Check sheet for the modelled part. Datum: model origin and axes. Units: mm. Round coordinates to 2 decimals unless told otherwise and drop trailing zeros. Write each loop counter-clockwise with the first axis right and the second up, starting at its lowest first coordinate (ties: lowest second). Pieces come first, ordered by that corner, then holes.
Item 1: Cross-section at A-A on x = -29. Enter the section's corners in (y, z), plus the area to 3 significant figures.
Item 2: Material ranges on line 1 (Z direction, x = 19, y = 0.75); line 2 (Z direction, x = -29, y = 0.35); line 3 (X direction, y = 0.7, z = 23), recorded low to high.
Item 3: Go/stop test with a flat-tipped pin: pin 1 Ø5 at (x, z) = (-29, -23) entering from +Y. Record where the tip stops, or that it passes through.
Item 4: Cross-section at B-B on x = 19. Enter the section's corners in (y, z), plus the area to 3 significant figures.
from build123d import *

# Parameters (mm, degrees)
SKETCH1_W                    = 85
SKETCH1_H                    = 56
BOSS_EXTRUDE1_DEPTH          = 3
M2_CLEARANCE_HOLE1_D         = 2.2
M2_CLEARANCE_HOLE1_DEPTH     = 5
M2_CLEARANCE_HOLE1_TIP       = 0.660946681
FILLET1_R                    = 3
CSK_FOR_M3_SFHCS1_AT_2_COUNT = 2
CSK_FOR_M3_SFHCS1_AT_2_PITCH = 74.027022093
CSK_FOR_M3_SFHCS1_AT_3_COUNT = 2
CSK_FOR_M3_SFHCS1_AT_3_PITCH = 46
CSK_FOR_M3_SFHCS1_AT_4_COUNT = 2
CSK_FOR_M3_SFHCS1_AT_4_PITCH = 58


with BuildPart() as part:
    # Sketch1 → Boss-Extrude1 (new body)
    with BuildSketch(Plane(origin=(0, 0, 0), x_dir=(1, 0, 0), z_dir=(0, 1, 0))):
        Rectangle(SKETCH1_W, SKETCH1_H)
    extrude(amount=BOSS_EXTRUDE1_DEPTH)

    # M2 Clearance Hole1
    with Locations(Plane(origin=(0, 3, 0), x_dir=(1, 0, 0), z_dir=(0, 1, 0))):
        with Locations((-39, 24.5), (19, -24.5), (19, 24.5), (-39, -24.5)):
            Hole(M2_CLEARANCE_HOLE1_D / 2, depth=M2_CLEARANCE_HOLE1_DEPTH)
            with Locations((0, 0, -(M2_CLEARANCE_HOLE1_DEPTH + M2_CLEARANCE_HOLE1_TIP / 2))):  # 118° drill point
                Cone(0, M2_CLEARANCE_HOLE1_D / 2, M2_CLEARANCE_HOLE1_TIP, mode=Mode.SUBTRACT)

    # Fillet1
    fillet1_edges = [part.edges().sort_by_distance(p)[0] for p in [
        (-42.5, 1.5, -28),
        (42.5, 1.5, -28),
        (42.5, 1.5, 28),
        (-42.5, 1.5, 28),
    ]]
    fillet(fillet1_edges, radius=FILLET1_R)

    # Sketch6 → CSK for M3 SFHCS1 (revolve, cut)
    with BuildSketch(Plane(origin=(-29, 3, -23), x_dir=(0, 0, 1), z_dir=(1, 0, 0))):
        Polygon((0, 0), (0, 3), (1.6, 3), (1.6, 1.76), (3.36, 0), align=None)
    csk_for_m3_sfhcs1 = revolve(axis=Axis((-29, 9.35, -23), (0, -1, 0)), mode=Mode.SUBTRACT)

    # CSK for M3 SFHCS1 at 2: CSK for M3 SFHCS1 ×2
    with Locations(*[Vector(0.7834976790895338, 0, 0.621394711002044) * (i * CSK_FOR_M3_SFHCS1_AT_2_PITCH) for i in range(1, CSK_FOR_M3_SFHCS1_AT_2_COUNT)]):
        add(csk_for_m3_sfhcs1, mode=Mode.SUBTRACT)

    # CSK for M3 SFHCS1 at 3: CSK for M3 SFHCS1 ×2
    with Locations(*[(0, 0, i * CSK_FOR_M3_SFHCS1_AT_3_PITCH) for i in range(1, CSK_FOR_M3_SFHCS1_AT_3_COUNT)]):
        add(csk_for_m3_sfhcs1, mode=Mode.SUBTRACT)

    # CSK for M3 SFHCS1 at 4: CSK for M3 SFHCS1 ×2
    with Locations(*[(i * CSK_FOR_M3_SFHCS1_AT_4_PITCH, 0, 0) for i in range(1, CSK_FOR_M3_SFHCS1_AT_4_COUNT)]):
        add(csk_for_m3_sfhcs1, mode=Mode.SUBTRACT)


solid = part.part
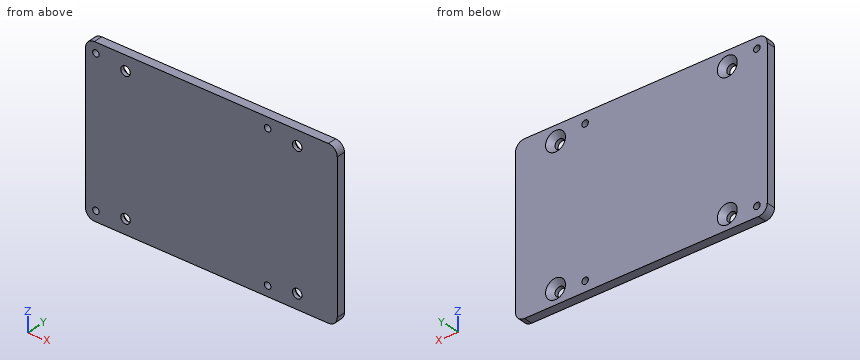
Response values:
1. outline: (0, -28) - (3, -28) - (3, -26.36) - (1.24, -24.6) - (0, -24.6) - close; (0, -21.4) - (1.24, -21.4) - (3, -19.64) - (3, 19.64) - (1.24, 21.4) - (0, 21.4) - close; (0, 24.6) - (1.24, 24.6) - (3, 26.36) - (3, 28) - (0, 28) - close
1. area: 143 mm2
2. line 1: z = -28 to -25.6, -23.4 to 23.4, 25.6 to 28
2. line 2: z = -28 to -24.6, -21.4 to 21.4, 24.6 to 28
2. line 3: x = -42.5 to -30.6, -27.4 to 27.4, 30.6 to 42.5
3. pin 1: stops at y = 2.14
4. outline: (0, -28) - (3, -28) - (3, -25.6) - (0, -25.6) - close; (0, -23.4) - (3, -23.4) - (3, 23.4) - (0, 23.4) - close; (0, 25.6) - (3, 25.6) - (3, 28) - (0, 28) - close
4. area: 155 mm2
